```python
from build123d import *

# Parameters (mm, degrees)
SKETCH1_W           = 50
SKETCH1_H           = 50
BOSS_EXTRUDE1_DEPTH = 123.5
SKETCH2_R           = 3.25
CUT_EXTRUDE1_DEPTH  = 50
SKETCH3_OUTSIDE_W   = 80.462
SKETCH3_OUTSIDE_H   = 80.462
SKETCH3_OUTSIDE_R   = 10
CUT_EXTRUDE2_DEPTH  = 123.5


with BuildPart() as part:
    # Sketch1 → Boss-Extrude1 (new body)
    with BuildSketch(Plane.XY):
        with Locations((2.064220183, 0.458715596)):
            Rectangle(SKETCH1_W, SKETCH1_H)
    extrude(amount=BOSS_EXTRUDE1_DEPTH)

    # Sketch2 → Cut-Extrude1 (cut)
    with BuildSketch(Plane.ZY.offset(22.935779817)):
        with Locations(Location((9.45, 0.458715596, 0), (0, 0, 270))):
            Circle(SKETCH2_R)
    extrude(amount=-CUT_EXTRUDE1_DEPTH, mode=Mode.SUBTRACT)

    # Sketch3 outside → Cut-Extrude2 (cut)
    with BuildSketch(Plane(origin=(0, 0, 0), x_dir=(-1, 0, 0), z_dir=(0, 0, -1))):
        with Locations((-2.064, 0.459)):
            Rectangle(SKETCH3_OUTSIDE_W, SKETCH3_OUTSIDE_H)
        with Locations((-2.064220183, 0.458715596)):
            Circle(SKETCH3_OUTSIDE_R, mode=Mode.SUBTRACT)
    extrude(amount=-CUT_EXTRUDE2_DEPTH, mode=Mode.SUBTRACT)


solid = part.part
```
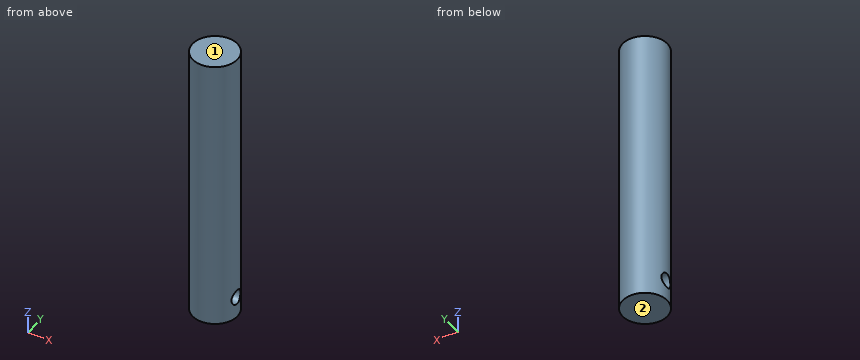
Verification items for the finished model (mm, model axes). Face numbers are marked on the shaded views. Give positions to 0.01 mm unless a question says otherwise; leave off trailing zeros. Order: outer loops, then holes, each group sorted by start corner. A loop starts at its lowest first (then second) coordinate and runs counter-clockwise, first axis right, second up. Notation, with made-up numbers: M 11.25,18 L 40.25,18 A22 cw 40.25,34 Z; hole C -38,-13.5 d7. An arc over 180 degrees is marked long. Return JSON: item names as keys, results as strings. Group by question number.
1) Section check B-B on x = 5.25. Record the cut outline in (y, z), and give its area (3 significant figures).
2) Go/stop test with flat-tipped pins: pin 1 Ø1.5 at (x, z) = (1, 51.5) entering from -Y; pin 2 Ø1 at (y, z) = (1.5, 35) entering from +X; pin 3 Ø5 at (x, y) = (5.5, 3) entering from -Z; pin 4 Ø1.5 at (x, z) = (-2, 45) entering from +Y. Record where each tip stops, or that it passes through.
3) Section check D-D on z = 53.5. Record the cut outline in (x, y), and give its area (3 significant figures).
4) Section check C-C on z = 10.5. Record the cut outline in (x, y), and give its area (3 significant figures).
5) Scan lines: line 1 (Z direction, x = 6.5, y = 0.75); line 2 (Y direction, x = 1.75, z = 9.45); line 3 (Y direction, x = 8.5, z = 9). Record each from-to range of solid material in increasing order.
6) Section check A-A on y = 1.5. Record the cut outline in (x, z).
7) Mould release check, pull along Z, two halves, no side actions. Record for the marked faces 1 and 2: pulls with the +Z half, pulls with the -Z half, needs draft (parallel to the pull), parting line crosses it, or undercut.
Answer block:
{
 "1": {"outline": "M -9.02,0 L 9.94,0 L 9.94,123.5 L -9.02,123.5 Z; hole C 0.46,9.45 d6.5", "area": "2,310 mm^2"},
 "2": {"pin 1": "stops at y = -9.54", "pin 2": "stops at x = 12.05", "pin 3": "stops at z = 0", "pin 4": "stops at y = 9.89"},
 "3": {"outline": "C 2.06,0.46 d20", "area": "314 mm^2"},
 "4": {"outline": "M -7.45,-2.62 A10 ccw 11.58,-2.62 Z; M -7.45,3.53 L 11.58,3.53 A10 ccw Z", "area": "193 mm^2"},
 "5": {"line 1": "z = 0 to 6.21, 12.69 to 123.5", "line 2": "y = -9.54 to -2.79, 3.71 to 10.45", "line 3": "y = -7.2 to -2.76, 3.68 to 8.11"},
 "6": {"outline": "M -7.88,0 L 12.01,0 L 12.01,6.37 L -7.88,6.37 Z; M -7.88,12.53 L 12.01,12.53 L 12.01,123.5 L -7.88,123.5 Z"},
 "7": {"face 1": "pulls with the +Z half", "face 2": "pulls with the -Z half"}
}
